from build123d import *

# Parameters (mm, degrees)
BOSS_EXTRUDE5_DEPTH = 2
CUT_EXTRUDE17_DEPTH = 2
SKETCH11_3_W        = 3
SKETCH11_3_H        = 3
CUT_EXTRUDE18_DEPTH = 2
CUT_EXTRUDE19_DEPTH = 2
SKETCH14_W          = 2.001486185
SKETCH14_H          = 2
CUT_EXTRUDE20_DEPTH = 2
SKETCH13_W          = 2.001486185
SKETCH13_H          = 2
CUT_EXTRUDE21_DEPTH = 2


with BuildPart() as part:
    # Sketch1 → Boss-Extrude5 (new body)
    with BuildSketch(Plane.XY):
        with BuildLine():
            Line((-22, 10), (-22, -10))
            Line((-22, -10), (-48.989794856, -10))
            ThreePointArc((-48.989794856, -10), (50, 0), (-48.989794856, 10))
            Line((-48.989794856, 10), (-22, 10))
        make_face()
    extrude(amount=-BOSS_EXTRUDE5_DEPTH)

    # Sketch11 → Cut-Extrude17 (cut)
    with BuildSketch(Plane(origin=(0, 0, -2), x_dir=(-1, 0, 0), z_dir=(0, 0, -1))):
        with BuildLine():
            Line((-1.5, 1.5), (1.5, 1.5))
            Line((1.5, 1.5), (1.5, 9.886859967))
            ThreePointArc((1.5, 9.886859967), (0, 10), (-1.5, 9.886859967))
            Line((-1.5, 9.886859967), (-1.5, 1.5))
        make_face()
    extrude(amount=-CUT_EXTRUDE17_DEPTH, mode=Mode.SUBTRACT)

    # Sketch11<3> → Cut-Extrude18 (cut)
    with BuildSketch(Plane(origin=(0, 0, -2), x_dir=(-1, 0, 0), z_dir=(0, 0, -1))):
        with BuildLine():
            Line((-9.886859967, -1.5), (-1.5, -1.5))
            Line((-1.5, -1.5), (-1.5, 1.5))
            Line((-1.5, 1.5), (-9.886859967, 1.5))
            ThreePointArc((-9.886859967, 1.5), (-10, 0), (-9.886859967, -1.5))
        make_face()
        with BuildLine():
            Line((1.5, 1.5), (1.5, -1.5))
            Line((1.5, -1.5), (9.886859967, -1.5))
            ThreePointArc((9.886859967, -1.5), (9.971674876, -0.752130419), (10, 0))
            ThreePointArc((10, 0), (9.971674876, 0.752130419), (9.886859967, 1.5))
            Line((9.886859967, 1.5), (1.5, 1.5))
        make_face()
        with BuildLine():
            Line((1.5, -9.886859967), (1.5, -1.5))
            Line((1.5, -1.5), (-1.5, -1.5))
            Line((-1.5, -1.5), (-1.5, -9.886859967))
            ThreePointArc((-1.5, -9.886859967), (0, -10), (1.5, -9.886859967))
        make_face()
        Rectangle(SKETCH11_3_W, SKETCH11_3_H)
    extrude(amount=-CUT_EXTRUDE18_DEPTH, mode=Mode.SUBTRACT)

    # Sketch1<9> → Cut-Extrude19 (cut)
    with BuildSketch(Plane.XY):
        with BuildLine():
            Line((32.494897428, 10), (22, 10))
            Line((22, 10), (22, -10))
            Line((22, -10), (48.989794856, -10))
            ThreePointArc((48.989794856, -10), (49.74680765, -5.0254481), (50, 0))
            ThreePointArc((50, 0), (49.74680765, 5.0254481), (48.989794856, 10))
            Line((48.989794856, 10), (32.494897428, 10))
        make_face()
    extrude(amount=-CUT_EXTRUDE19_DEPTH, mode=Mode.SUBTRACT)

    # Sketch14 → Cut-Extrude20 (cut)
    with BuildSketch(Plane.ZY.offset(22)):
        with Locations((-0.999256907, -5.028117734)):
            Rectangle(SKETCH14_W, SKETCH14_H)
        with Locations((-0.999256907, 4.972809543)):
            Rectangle(SKETCH14_W, SKETCH14_H)
    extrude(amount=-CUT_EXTRUDE20_DEPTH, mode=Mode.SUBTRACT)

    # Sketch13 → Cut-Extrude21 (cut)
    with BuildSketch(Plane(origin=(22, 0, 0), x_dir=(0, 0, -1), z_dir=(1, 0, 0))):
        with Locations((0.999256907, -5.028117734)):
            Rectangle(SKETCH13_W, SKETCH13_H)
        with Locations((0.999256907, 4.972809543)):
            Rectangle(SKETCH13_W, SKETCH13_H)
    extrude(amount=-CUT_EXTRUDE21_DEPTH, mode=Mode.SUBTRACT)


solid = part.part
The listing builds one solid part. Answer for the finished solid, in the listing's coordinates (mm). Coordinates: 2 decimals unless noted, no trailing zeros. Write each loop counter-clockwise with the first axis right and the second up, starting at its lowest first coordinate (ties: lowest second). Pieces come first, ordered by that corner, then holes. Notation, with made-up numbers: (43, 82.25) - (65, 82.25) arc R19 cw to (65, 106.25) - close; hole circle Ø5 at (1, 8). An arc over 180 degrees is marked (long way). Put each result on its own line as item: value.
1. Flat-ended cylindrical pins translate along their axes: pin 1 Ø6 at (x, y) = (-30.5, 11) entering from +Z; pin 2 Ø0.6 at (y, z) = (-5, -1) entering from +X; pin 3 Ø1 at (x, z) = (4, -0.5) entering from +Y; pin 4 Ø1 at (y, z) = (6, -1) entering from -X. Find the tip coordinate at first contact, or state that the pin passes through.
Answer sheet:
pin 1: stops at z = 0
pin 2: stops at x = 20
pin 3: stops at y = 49.88
pin 4: stops at x = -22
2. The part is cut by section C-C on x = -13. Give the vertices of the cut face in (y, z), plus the area to 3 significant figures.
Answer sheet:
outline: (-48.28, -2) - (48.28, -2) - (48.28, 0) - (-48.28, 0) - close
area: 193 mm^2
3. Find the intervals of material crossed by line 1 along X through (y, z) = (0, -0.65); line 2 along X through (y, z) = (-8, -0.45); line 3 along Y through (x, z) = (6.5, -0.7), in increasing order. Write a range as from..to.
Answer sheet:
line 1: x = -22..-10, 10..22
line 2: x = -22..-1.5, 1.5..22
line 3: y = -49.58..-1.5, 1.5..49.58
4. The part is cut by section A-A on x = -36.5. Give the vertices of the cut face in (y, z), plus the area to 3 significant figures.
Answer sheet:
outline: (-34.17, -2) - (-10, -2) - (-10, 0) - (-34.17, 0) - close; (10, -2) - (34.17, -2) - (34.17, 0) - (10, 0) - close
area: 96.7 mm^2
5. The part is cut by section B-B on y = -42. Give the vertices of the cut face in (x, z).
Answer sheet:
outline: (-27.13, -2) - (27.13, -2) - (27.13, 0) - (-27.13, 0) - close
6. Determine the mould class of faces 1 (the face through (10.2, 0.7, -2)), 2 (the face through (-0.96, -49.99, -0.99)) for opening direction X: pulls with the +X half, pulls with the -X half, needs draft (parallel to the pull), parting line crosses it, or undercut.
Answer sheet:
face 1: needs draft
face 2: parting line crosses it
